Geometry check sheet. Reference: the model listing, model coordinates, mm. A direction names the side the tool comes from. Round coordinates to 2 decimals unless told otherwise and drop trailing zeros. Loops run counter-clockwise (first coordinate to the right, second up) from the corner with the lowest first, then second, coordinate; pieces in that order, holes last.
```python
from build123d import *

# Parameters (mm, degrees)
SKETCH1_W                        = 15
SKETCH1_H                        = 6
MAIN_BODY_EXT_DEPTH              = 8.3
EMISSION_PATH_EXT_DEPTH          = 9
SKETCH3_R                        = 1.25
EMISSION_AND_GRIN_CUT_DEPTH      = 20.092931
SKETCH4_R                        = 1
DRUM_LENS_CUT_DEPTH              = 13
SKETCH41_R                       = 1
ADDTL_LIGHT_SOURCE_DEPTH         = 5
SKETCH5_W                        = 15
SKETCH5_H                        = 7.3
FILTERCOVER_CUT1_DEPTH           = 1
TOP_LED_SCREW_W                  = 3.06
TOP_LED_SCREW_H                  = 2
BOSS_EXTRUDE1_DEPTH              = 1
FILTERSET_CUT2_DEPTH             = 4
SKETCH10_R                       = 2.5
EMISSION_LENS_CUT_DEPTH          = 8.5
SKETCH15_R                       = 0.795
MAGNETS_CUT_DEPTH                = 0.9
SCREW_HOLES_CUT_DEPTH            = 20.507434
SCREW_HOLES_CUT_DEPTH_BACK       = 2.5
SKETCH18_R                       = 0.375
EXTERNAL_FILLET_1_R              = 1.5
VERTICAL_PATH_CUT_DEPTH          = 14.011149
VERTICAL_PATH_CUT_DEPTH_BACK     = 4
SKETCH28_R                       = 1.5
CUT_EXTRUDE_ORIGINAL_LIGHT_DEPTH = 0.7
CUT_EXTRUDE_ADDTL_LIGHT_DEPTH    = 0.7
SKETCH29_R                       = 0.375
SIDE_LED_SCREW_DEPTH             = 2.5
SKETCH32_W                       = 2
SKETCH32_H                       = 2.36
SIDE_WIRE_SLOT_CUT_DEPTH         = 0.7
SKETCH45_W                       = 2.36
SKETCH45_H                       = 2
TOP_LED_SLOT_DEPTH               = 0.7
CUT_EXTRUDE16_DEPTH              = 9
CUT_EXTRUDE17_REACH              = 13.945
SKETCH37_R                       = 2
SKETCH51_R                       = 0.375
TOP_LE_SCREW_DEPTH               = 2.1
NOTCH_EXTRUDE_DEPTH              = 2


with BuildPart() as part:
    # Sketch1 → Main Body Ext (new body)
    with BuildSketch(Plane(origin=(0, 0, 0), x_dir=(1, 0, 0), z_dir=(0, 1, 0))):
        Rectangle(SKETCH1_W, SKETCH1_H)
    extrude(amount=MAIN_BODY_EXT_DEPTH)

    # Sketch8 → Emission Path Ext (add)
    with BuildSketch(Plane(origin=(0, 8.3, 0), x_dir=(1, 0, 0), z_dir=(0, 1, 0))):
        Polygon((-2.75, 3), (-1.5, 1.75), (-1.5, -3), (-7.5, -3), (-7.5, 3), align=None)
    extrude(amount=EMISSION_PATH_EXT_DEPTH)

    # Sketch3 → Emission and Grin Cut (cut, through all)
    with BuildSketch(Plane.XZ):
        with Locations(Location((-4.5, 0, 0), (0, 0, 270))):
            Circle(SKETCH3_R)
    extrude(amount=-EMISSION_AND_GRIN_CUT_DEPTH, mode=Mode.SUBTRACT)

    # Sketch4 → Drum Lens Cut (cut)
    with BuildSketch(Plane(origin=(7.5, 0, 0), x_dir=(0, 0, -1), z_dir=(1, 0, 0))):
        with Locations((0, 3)):
            Circle(SKETCH4_R)
    extrude(amount=-DRUM_LENS_CUT_DEPTH, mode=Mode.SUBTRACT)

    # Sketch41 → Addtl Light Source (cut)
    with BuildSketch(Plane(origin=(0, 8.3, 0), x_dir=(1, 0, 0), z_dir=(0, 1, 0))):
        with Locations(Location((1.5, 0, 0), (0, 0, 270))):
            Circle(SKETCH41_R)
    extrude(amount=-ADDTL_LIGHT_SOURCE_DEPTH, mode=Mode.SUBTRACT)

    # Sketch5 → FilterCover Cut1 (cut)
    with BuildSketch(Plane.XY.offset(3)):
        with Locations((0, 4.65)):
            Rectangle(SKETCH5_W, SKETCH5_H)
    extrude(amount=-FILTERCOVER_CUT1_DEPTH, mode=Mode.SUBTRACT)

    # Top-LED-Screw → Boss-Extrude1 (add)
    with BuildSketch(Plane.XY.offset(2)):
        with Locations((5.97, 7.3)):
            Rectangle(TOP_LED_SCREW_W, TOP_LED_SCREW_H)
    extrude(amount=BOSS_EXTRUDE1_DEPTH)

    # Sketch6 → FilterSet Cut2 (cut)
    with BuildSketch(Plane.XY.offset(2)):
        with BuildLine():
            Line((5.3, 4.5), (5.3, 1.8))
            ThreePointArc((5.3, 1.8), (5.7, 1.4), (5.3, 1))
            Line((5.3, 1), (4.1, 1))
            ThreePointArc((4.1, 1), (3.7, 1.4), (4.1, 1.8))
            Line((4.1, 1.8), (4.1, 4.5))
            ThreePointArc((4.1, 4.5), (4.7, 5.1), (5.3, 4.5))
        make_face()
        with BuildLine():
            Line((-6.9, 7.9), (-6.9, 7.5))
            ThreePointArc((-6.9, 7.5), (-6.782843, 7.217157), (-6.5, 7.1))
            Line((-6.5, 7.1), (-2.5, 7.1))
            ThreePointArc((-2.5, 7.1), (-2.217157, 7.217157), (-2.1, 7.5))
            Line((-2.1, 7.5), (-2.1, 7.9))
            ThreePointArc((-2.1, 7.9), (-2.217157, 8.182843), (-2.5, 8.3))
            Line((-2.5, 8.3), (-6.5, 8.3))
            ThreePointArc((-6.5, 8.3), (-6.782843, 8.182843), (-6.9, 7.9))
        make_face()
        with BuildLine():
            Line((-2.605887, 6.591169), (-6.848528, 2.348528))
            ThreePointArc((-6.848528, 2.348528), (-6.848528, 1.5), (-6, 1.5))
            Line((-6, 1.5), (-1.757359, 5.742641))
            ThreePointArc((-1.757359, 5.742641), (-1.757359, 6.591169), (-2.605887, 6.591169))
        make_face()
        with BuildLine():
            Line((3.112092, 6.591169), (-1.130548, 2.348528))
            ThreePointArc((-1.130548, 2.348528), (-1.130548, 1.5), (-0.28202, 1.5))
            Line((-0.28202, 1.5), (3.96062, 5.742641))
            ThreePointArc((3.96062, 5.742641), (3.96062, 6.591169), (3.112092, 6.591169))
        make_face()
    extrude(amount=-FILTERSET_CUT2_DEPTH, mode=Mode.SUBTRACT)

    # Sketch10 → Emission Lens Cut (cut)
    with BuildSketch(Plane(origin=(0, 17.3, 0), x_dir=(1, 0, 0), z_dir=(0, 1, 0))):
        with Locations(Location((-4.5, 0, 0), (0, 0, 270))):
            Circle(SKETCH10_R)
    extrude(amount=-EMISSION_LENS_CUT_DEPTH, mode=Mode.SUBTRACT)

    # Sketch15 → Magnets Cut (cut)
    with BuildSketch(Plane.XZ):
        with Locations(Location((-6.25, -1.875, 0), (0, 0, 270))):
            Circle(SKETCH15_R)
        with Locations(Location((-6.25, 1.875, 0), (0, 0, 270))):
            Circle(SKETCH15_R)
        with Locations(Location((-1.5, 0, 0), (0, 0, 270))):
            Circle(SKETCH15_R)
    extrude(amount=-MAGNETS_CUT_DEPTH, mode=Mode.SUBTRACT)

    # Sketch18 → Screw Holes Cut (cut, two sides: drawn at the far end of the back side and taken through both)
    with BuildSketch(Plane.XY.offset(2).offset(-SCREW_HOLES_CUT_DEPTH_BACK)):
        with Locations(Location((-6.5, 4, 0), (0, 0, 180))):
            Circle(SKETCH18_R)
        with Locations(Location((6, 5.8, 0), (0, 0, 180))):
            Circle(SKETCH18_R)
        with Locations((0.25, 1)):
            Circle(SKETCH18_R)
    extrude(amount=SCREW_HOLES_CUT_DEPTH + SCREW_HOLES_CUT_DEPTH_BACK, mode=Mode.SUBTRACT)

    # External Fillet 1
    # the kernel refuses this fillet: 1.5 mm, written as the material it takes off along each edge
    with BuildSketch(Plane(origin=(-7.5, -3.75, -3), x_dir=(1, 0, 0), z_dir=(0, 1, 0))) as external_fillet_1_piece_1:
        with BuildLine():
            CenterArc((EXTERNAL_FILLET_1_R, -EXTERNAL_FILLET_1_R), EXTERNAL_FILLET_1_R, 90, 90)
            Line((0, -EXTERNAL_FILLET_1_R), (0, 0))
            Line((0, 0), (EXTERNAL_FILLET_1_R, 0))
        make_face()
    extrude(amount=24.8, mode=Mode.SUBTRACT)
    with BuildSketch(Plane(origin=(-1.5, 8.3, 3), x_dir=(0, 0, -1), z_dir=(0, 1, 0))) as external_fillet_1_piece_2:
        with BuildLine():
            CenterArc((EXTERNAL_FILLET_1_R, EXTERNAL_FILLET_1_R), EXTERNAL_FILLET_1_R, 180, 90)
            Line((0, EXTERNAL_FILLET_1_R), (0, 0))
            Line((0, 0), (EXTERNAL_FILLET_1_R, 0))
        make_face()
    extrude(amount=12.75, mode=Mode.SUBTRACT)

    # Sketch28 → Vertical-Path-Cut (cut, two sides: drawn at the far end of the back side and taken through both)
    with BuildSketch(Plane(origin=(0, 7.1, 0), x_dir=(1, 0, 0), z_dir=(0, 1, 0)).offset(-VERTICAL_PATH_CUT_DEPTH_BACK)):
        with Locations(Location((-4.5, 0, 0), (0, 0, 180))):
            Circle(SKETCH28_R)
    extrude(amount=VERTICAL_PATH_CUT_DEPTH + VERTICAL_PATH_CUT_DEPTH_BACK, mode=Mode.SUBTRACT)

    # Sketch12 → Cut-Extrude Original Light (cut)
    with BuildSketch(Plane(origin=(7.5, 0, 0), x_dir=(0, 0, -1), z_dir=(1, 0, 0))):
        with BuildLine():
            Line((1.6, 5.94), (-1.6, 5.94))
            Line((-1.6, 5.94), (-2, 5.94))
            Line((-2, 5.94), (-2, 1.33))
            Line((-2, 1.33), (1.6, 1.33))
            ThreePointArc((1.6, 1.33), (1.882843, 1.447157), (2, 1.73))
            Line((2, 1.73), (2, 5.54))
            ThreePointArc((2, 5.54), (1.882843, 5.822843), (1.6, 5.94))
        make_face()
    extrude(amount=-CUT_EXTRUDE_ORIGINAL_LIGHT_DEPTH, mode=Mode.SUBTRACT)

    # Sketch44 → Cut-Extrude Addtl Light (cut)
    with BuildSketch(Plane(origin=(0, 8.3, 0), x_dir=(1, 0, 0), z_dir=(0, 1, 0))):
        with BuildLine():
            Line((-0.17, -2), (4.44, -2))
            Line((4.44, -2), (4.44, 1.6))
            ThreePointArc((4.44, 1.6), (4.322843, 1.882843), (4.04, 2))
            Line((4.04, 2), (0.23, 2))
            ThreePointArc((0.23, 2), (-0.052843, 1.882843), (-0.17, 1.6))
            Line((-0.17, 1.6), (-0.17, -2))
        make_face()
    extrude(amount=-CUT_EXTRUDE_ADDTL_LIGHT_DEPTH, mode=Mode.SUBTRACT)

    # Sketch29 → Side-LED-Screw (cut)
    with BuildSketch(Plane(origin=(7.5, 0, 0), x_dir=(0, 0, -1), z_dir=(1, 0, 0))):
        with Locations((2, 6.5)):
            Circle(SKETCH29_R)
    extrude(amount=-SIDE_LED_SCREW_DEPTH, mode=Mode.SUBTRACT)

    # Sketch32 → Side-Wire-Slot-Cut (cut)
    with BuildSketch(Plane(origin=(7.5, 0, 0), x_dir=(0, 0, -1), z_dir=(1, 0, 0))):
        with Locations((0, 7.12)):
            Rectangle(SKETCH32_W, SKETCH32_H)
    extrude(amount=-SIDE_WIRE_SLOT_CUT_DEPTH, mode=Mode.SUBTRACT)

    # Sketch45 → Top-LED-slot (cut)
    with BuildSketch(Plane(origin=(0, 8.3, 0), x_dir=(1, 0, 0), z_dir=(0, 1, 0))):
        with Locations((5.62, 0)):
            Rectangle(SKETCH45_W, SKETCH45_H)
    extrude(amount=-TOP_LED_SLOT_DEPTH, mode=Mode.SUBTRACT)

    # Sketch33 → Side-BallLens_Cut (revolve, cut)
    with BuildSketch(Plane.XY, mode=Mode.PRIVATE) as side_balllens_cut_sk:
        with BuildLine():
            Line((6.8, 3), (5.3, 3))
            ThreePointArc((5.3, 3), (5.73934, 4.06066), (6.8, 4.5))
            Line((6.8, 4.5), (6.8, 3))
        make_face()
    revolve(side_balllens_cut_sk.sketch.rotate(Axis((6.8, 3, 0), (-1, 0, 0)), 84.26086), axis=Axis((6.8, 3, 0), (-1, 0, 0)), mode=Mode.SUBTRACT)

    # Sketch47 → Top-BallLens_Cut (revolve, cut)
    with BuildSketch(Plane(origin=(1.5, 0, 0), x_dir=(0, 0, -1), z_dir=(1, 0, 0))):
        with BuildLine():
            Line((-1.5, 7.6), (0, 7.6))
            Line((0, 7.6), (0, 6.137287))
            ThreePointArc((0, 6.137287), (-1.04756, 6.563498), (-1.5, 7.6))
        make_face()
    revolve(axis=Axis((1.5, 7.6, 0), (0, -1, 0)), mode=Mode.SUBTRACT)

    # Sketch36 → Cut-Extrude16 (cut)
    with BuildSketch(Plane(origin=(0, 17.3, 0), x_dir=(1, 0, 0), z_dir=(0, 1, 0))):
        with BuildLine():
            Line((-7.5, -1.5), (-7.5, -3))
            Line((-7.5, -3), (-6, -3))
            ThreePointArc((-6, -3), (-7.06066, -2.56066), (-7.5, -1.5))
        make_face()
    extrude(amount=-CUT_EXTRUDE16_DEPTH, mode=Mode.SUBTRACT)

    # Sketch37 → Cut-Extrude17 (cut, up to next)
    with BuildSketch(Plane(origin=(0, 8.8, 0), x_dir=(1, 0, 0), z_dir=(0, 1, 0)), mode=Mode.PRIVATE) as cut_extrude17_sk1:
        with Locations(Location((-4.5, 0, 0), (0, 0, 180))):
            Circle(SKETCH37_R)
    cut_extrude17_tool1 = extrude(cut_extrude17_sk1.sketch, amount=-CUT_EXTRUDE17_REACH, mode=Mode.PRIVATE) & part.part
    add(cut_extrude17_tool1.solids().sort_by_distance((-4.5, 8.8, 0))[0], mode=Mode.SUBTRACT)

    # Sketch51 → Top-LE-Screw (cut)
    with BuildSketch(Plane(origin=(0, 8.3, 0), x_dir=(1, 0, 0), z_dir=(0, 1, 0))):
        with Locations(Location((5, -2, 0), (0, 0, 270))):
            Circle(SKETCH51_R)
    extrude(amount=-TOP_LE_SCREW_DEPTH, mode=Mode.SUBTRACT)

    # Notch → Notch-Extrude (cut)
    with BuildSketch(Plane.XZ):
        Polygon((3.060555, -2.0476), (1.884933, -2.0476), (1.884933, -3), (4.489155, -3), align=None)
        Polygon((1.884933, -3), (1.884933, -2.0476), (1.25, -3), align=None)
    extrude(amount=-NOTCH_EXTRUDE_DEPTH, mode=Mode.SUBTRACT)


solid = part.part
```
1) Sectioned sample at A-A, the plane y = 10. Record the cut outline in (x, z), then the cut area to 3 significant figures.
Report:
outline: (-7.5, -1.5) arc R1.5 ccw to (-6, -3) - (-2.75, -3) - (-1.5, -1.75) - (-1.5, 1.5) arc R1.5 ccw to (-3, 3) - (-6, 3) arc R1.5 ccw to (-7.5, 1.5) - close; hole circle Ø5 at (-4.5, 0)
area: 14.1 mm2
2) Sectioned sample at B-B, the plane x = 6. State how many separate pieces and enclosed holes the cut face has, then the cut area to 3 significant figures.
Report:
separate pieces: 1
enclosed holes: 2
area: 35.7 mm2
3) Scan lines: line 1 along X through (y, z) = (6, 1.15); line 2 along X through (y, z) = (5.25, -1.1); line 3 along X through (y, z) = (1.25, 1.35). Record each from-to range of solid material in increasing order.
Report:
line 1: x = -7.5 to -5.46, -3.54 to -3.2, -1.61 to 2.52, 4.11 to 5.68, 6.32 to 7.5
line 2: x = -7.5 to -5.52, -2.25 to 1.77, 3.47 to 6.8
line 3: x = -7.5 to -0.03, 0.53 to 3.73, 5.67 to 7.5
4) Access from +Z, -Z, +X, -X, +Y, -Y to the whole of each face (thin tool, end or side, straight path). Record for faces 4 (the face through (-5.886, 5.555, -0.575)), 5 (the face through (-1.5, 13, 0)), 6 (the face through (3, 2, 0)), 7 (the face through (-6.1, 8.3, -1.5)).
Report:
face 4: +Y
face 5: +Z, -Z, +X, +Y
face 6: +X
face 7: +Z
5) Gauge pin test, flat ends, axial feed: pin 1 (1.2 mm diameter, centred on y = 3, z = 0, fed in from +X); pin 2 (1 mm diameter, centred on x = 6, z = 2.5, fed in from +Y); pin 3 (0.6 mm diameter, centred on x = 7.5, z = 0, fed in from +Y). Record the tip position at first contact, or that the pin passes through.
Report:
pin 1: stops at x = -5.91
pin 2: stops at y = 8.3
pin 3: stops at y = 1.33
6) Mould release check, pull along Y, two halves, no side actions. Record for faces 1 (the face through (-6, 0.9, -2)), 2 (the face through (-7.05, 8.53, -2.57)), 3 (the face through (5.7, 1.4, 0)): +Y half, -Y half, draft (parallel to the pull), parting line (faces both ways), or undercut.
Report:
face 1: -Y half
face 2: draft
face 3: undercut
